```python
from build123d import *

# Parameters (mm, degrees)
BASE_LINK_OUTLINE_R     = 5
BASE_LINK_OUTLINE_R_2   = 4
BASE_LINK_DEPTH         = 60
SKETCH3_R               = 4
BOSS_EXTRUDE1_DEPTH     = 60
BOSS_EXTRUDE2_DEPTH     = 4
CUT_EXTRUDE1_DEPTH      = 78.510329968
CUT_EXTRUDE1_DEPTH_BACK = 78.510329968
SKETCH5_R               = 2.5


# Read off the part's stored shape, not the designer's step: base_link
with BuildPart() as part:
    # base_link outline → base_link (new body)
    with BuildSketch(Plane(origin=(0, 0, 0), x_dir=(1, 0, 0), z_dir=(0, 1, 0))):
        with Locations((30.34635, 52.561420024)):
            Circle(BASE_LINK_OUTLINE_R)
        with Locations((30.34635, 52.561420024)):
            Circle(BASE_LINK_OUTLINE_R_2, mode=Mode.SUBTRACT)
    extrude(amount=BASE_LINK_DEPTH)


with BuildPart() as body_2:
    # Sketch3 → Boss-Extrude1 (new body)
    with BuildSketch(Plane(origin=(0, 0, 0), x_dir=(1, 0, 0), z_dir=(0, 1, 0))):
        with Locations(Location((30.34635, 52.561420024, 0), (0, 0, 270))):
            Circle(SKETCH3_R)
    extrude(amount=BOSS_EXTRUDE1_DEPTH)

    # Sketch4 → Boss-Extrude2 (add, symmetric)
    with BuildSketch(Plane(origin=(0, 0, 0), x_dir=(-0.49999999999999994, 0, 0.8660254037844387), z_dir=(-0.8660254037844386, 0, -0.4999999999999999))):
        with BuildLine():
            Line((-68.6927, 75), (-65.6927, 75))
            Line((-65.6927, 75), (-65.6927, 64))
            ThreePointArc((-65.6927, 64), (-65.399806781, 63.292893219), (-64.6927, 63))
            Line((-64.6927, 63), (-56.6927, 63))
            ThreePointArc((-56.6927, 63), (-55.985593219, 63.292893219), (-55.6927, 64))
            Line((-55.6927, 64), (-55.6927, 75))
            Line((-55.6927, 75), (-52.6927, 75))
            Line((-52.6927, 75), (-52.6927, 64))
            ThreePointArc((-52.6927, 64), (-53.864272875, 61.171572875), (-56.6927, 60))
            Line((-56.6927, 60), (-64.6927, 60))
            ThreePointArc((-64.6927, 60), (-67.521127125, 61.171572875), (-68.6927, 64))
            Line((-68.6927, 64), (-68.6927, 75))
        make_face()
    extrude(amount=BOSS_EXTRUDE2_DEPTH, both=True)

    # Sketch5 → Cut-Extrude1 (cut, two sides: drawn at the far end of the back side and taken through both)
    with BuildSketch(Plane(origin=(34.34635, 0, -59.489623255), x_dir=(-0.8660254037844386, 0, -0.5), z_dir=(0.5000000000000001, 0, -0.8660254037844387)).offset(-CUT_EXTRUDE1_DEPTH_BACK)):
        with Locations((0, 71)):
            Circle(SKETCH5_R)
        with BuildLine():
            Line((-4, 71), (-4, 76))
            Line((-4, 76), (4, 76))
            Line((4, 76), (4, 71))
            ThreePointArc((4, 71), (0, 75), (-4, 71))
        make_face()
    extrude(amount=CUT_EXTRUDE1_DEPTH + CUT_EXTRUDE1_DEPTH_BACK, mode=Mode.SUBTRACT)


solid = body_2.part
```
Verification items for the finished model (mm, model axes). A direction names the side the tool comes from. Round coordinates to 2 decimals unless told otherwise and drop trailing zeros. Loops run counter-clockwise (first coordinate to the right, second up) from the corner with the lowest first, then second, coordinate; pieces in that order, holes last. Notation, with made-up numbers: (22.5, 50) -> (41.5, 50) arc R18 ccw to (41.5, 85) -> close; hole circle Ø6 at (-5.5, 81.5). An arc over 180 degrees is marked (long way). Answer as a JSON object with one key per item and string values.
Q1. Scan lines: line 1 (X direction, y = 14, z = -52.75); line 2 (Z direction, x = 30.5, y = 17); line 3 (Y direction, x = 29.25, z = -54.25). Record each from-to range of solid material in increasing order. Write a range as from..to.
Data:
{"line 1": "x = 26.35..34.34", "line 2": "z = -56.56..-48.56", "line 3": "y = 0..63"}
Q2. Section check A-A (z = -52.75). Record the boundary of the cut face in (x, y), then the cut area to 3 significant figures.
Data:
{"outline": "(25.84, 60) -> (26.35, 60) -> (26.35, 0) -> (34.34, 0) -> (34.34, 60) -> (35.07, 60) -> (35.07, 63) -> (25.84, 63) -> close", "area": "507 mm2"}
Q3. Go/stop test with flat-tipped pins: P1, Ø3, axis at x = 30, y = 52, coming from the +Z side; P2, Ø2, axis at y = 55.5, z = -49, coming from the -X side; P3, Ø2, axis at x = 34.5, y = 18.5, coming from the +Z side. Record where each tip stops, or that it passes through.
Data:
{"P1": "stops at z = -48.56", "P2": "stops at x = 27.27", "P3": "stops at z = -50.1"}
Q4. Draft check along Y on faces 4 (the flat face through (35, 60, -54)), 5 (the flat face through (33.75, 61.91, -50.46)), 6 (the cylindrical face through (33.5, 75, -58.2)), 7 (the cylindrical face through (34.06, 68.56, -57.9)). Enter one of: pulls with the +Y half, pulls with the -Y half, needs draft (parallel to the pull), parting line crosses it, or undercut.
Data:
{"face 4": "pulls with the -Y half", "face 5": "needs draft", "face 6": "pulls with the +Y half", "face 7": "undercut"}
Q5. Section check B-B (y = 14.5). Record the boundary of the cut face in (x, z).
Data:
{"outline": "circle Ø8 at (30.35, -52.56)"}
Q6. Access from +Z, -Z, +X, -X, +Y, -Y to the whole of each face (thin tool, end or side, straight path). Record for faces 1 (the cylindrical face through (27.948, 63.285, -48.52)), 2 (the cylindrical face through (28.81, 29.58, -48.87)), 3 (the cylindrical face through (32.66, 63.3, -56.67)).
Data:
{"face 1": "+X, +Y", "face 2": "-Y", "face 3": "-X, +Y"}
